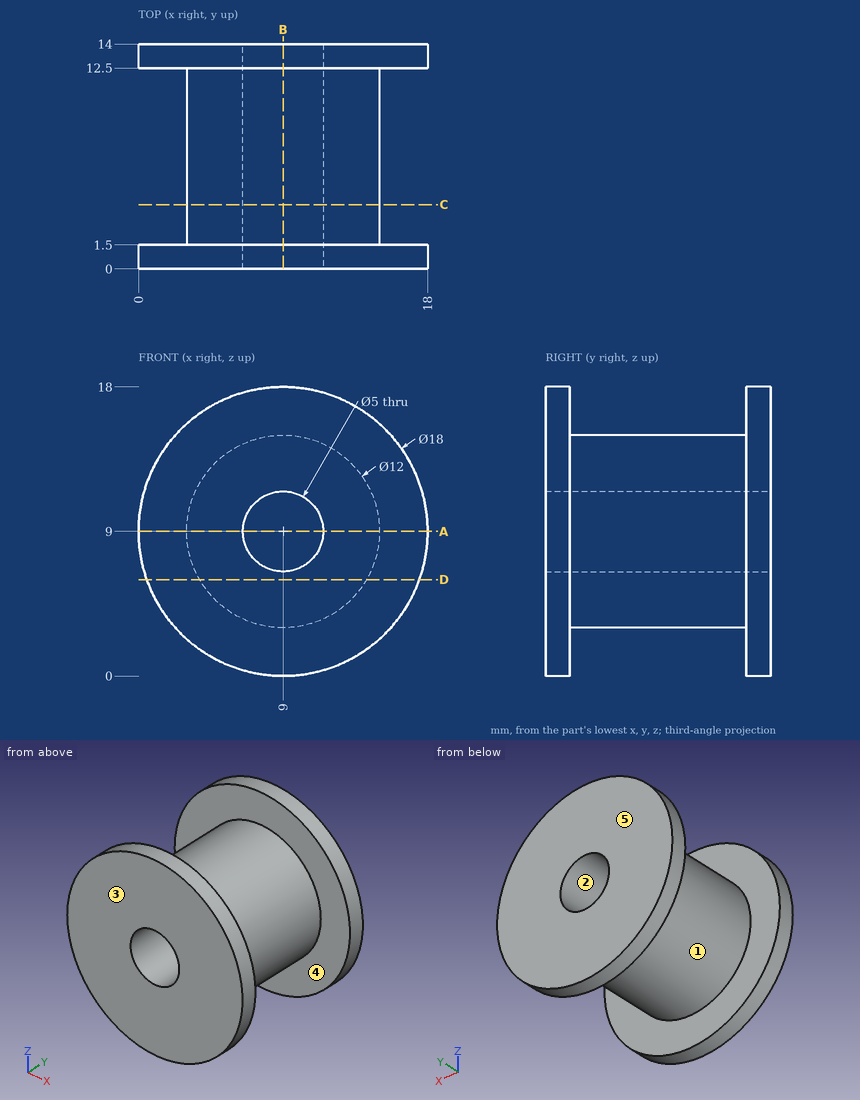
The figure shows three views and two pictorial views of one solid part (mm, origin at its lowest corner). Answer the questions. A direction names the side the tool comes from. Round coordinates to 2 decimals unless told otherwise and drop trailing zeros. Write each loop counter-clockwise with the first axis right and the second up, starting at its lowest first coordinate (ties: lowest second). Pieces come first, ordered by that corner, then holes. Notation, with made-up numbers: (45.25, 65) - (66.25, 65) arc R18 cw to (66.25, 84) - close; hole circle Ø2 at (-21.75, 34.25). An arc over 180 degrees is marked (long way). Use one line per item in the form item = value. Start each with the question number.
Item 1: Determine the mould class of the marked faces 1, 2 and 3 for opening direction Z: +Z half, -Z half, draft (parallel to the pull), parting line (faces both ways), or undercut.
Item 2: Find the intervals of material crossed by line 1 (Y direction, x = 4.75, z = 14.5); line 2 (X direction, y = 5.5, z = 9), in increasing order. Write a range as [from, to].
Item 3: A cutting plane is placed at D-D (z = 6). Write down the section's boundary in (x, y).
Item 4: A cutting plane is placed at C-C (y = 4). Write down the section's boundary in (x, z), plus the area to 3 significant figures.
Item 5: A cutting plane is placed at B-B (x = 9). Write down the section's boundary in (y, z).
Item 6: Flat-ended cylindrical pins translate along their axes: pin 1 Ø6 at (y, z) = (7.5, 8.5) entering from +X; pin 2 Ø2 at (x, y) = (13, 11) entering from -Z; pin 3 Ø4 at (x, y) = (9, 9) entering from -Z. Find the tip coordinate at first contact, or state that the pin passes through.
Item 7: A cutting plane is placed at A-A (z = 9). Write down the section's boundary in (x, y).
Item 8: A tool of negligible diameter and unlimited length cuts with its end or side. For the marked faces 4 and 5, from which of +Z, -Z, +X, -X, +Y, -Y can it reach the whole face along a straight path? Write none if from no direction.
The answers:
q1.face_1 = parting line
q1.face_2 = undercut
q1.face_3 = draft
q2.line_1 = [0, 1.5], [12.5, 14]
q2.line_2 = [3, 6.5], [11.5, 15]
q3.outline = (0.51, 0) - (17.49, 0) - (17.49, 1.5) - (14.2, 1.5) - (14.2, 12.5) - (17.49, 12.5) - (17.49, 14) - (0.51, 14) - (0.51, 12.5) - (3.8, 12.5) - (3.8, 1.5) - (0.51, 1.5) - close
q4.outline = circle Ø12 at (9, 9); hole circle Ø5 at (9, 9)
q4.area = 93.5 mm^2
q5.outline = (0, 0) - (1.5, 0) - (1.5, 3) - (12.5, 3) - (12.5, 0) - (14, 0) - (14, 6.5) - (0, 6.5) - close; (0, 11.5) - (14, 11.5) - (14, 18) - (12.5, 18) - (12.5, 15) - (1.5, 15) - (1.5, 18) - (0, 18) - close
q6.pin_1 = 15
q6.pin_2 = 3.8
q6.pin_3 = 3
q7.outline = (0, 0) - (6.5, 0) - (6.5, 14) - (0, 14) - (0, 12.5) - (3, 12.5) - (3, 1.5) - (0, 1.5) - close; (11.5, 0) - (18, 0) - (18, 1.5) - (15, 1.5) - (15, 12.5) - (18, 12.5) - (18, 14) - (11.5, 14) - close
q8.face_4 = none
q8.face_5 = +Z, -Z, +X, -X, +Y
